The drawing under review shows one solid part. Ordinate dimensions are in mm from its lowest x, y, z. A direction names the side the tool comes from. Give positions to 0.01 mm unless a question says otherwise; leave off trailing zeros. Write each loop counter-clockwise with the first axis right and the second up, starting at its lowest first coordinate (ties: lowest second). Pieces come first, ordered by that corner, then holes. Notation, with made-up numbers: (60, 66.25) -> (65, 66.25) arc R14 ccw to (65, 91.25) -> close; hole circle Ø10 at (44, 23). An arc over 180 degrees is marked (long way). Use CSV: the item, a comma, the result in double quotes.
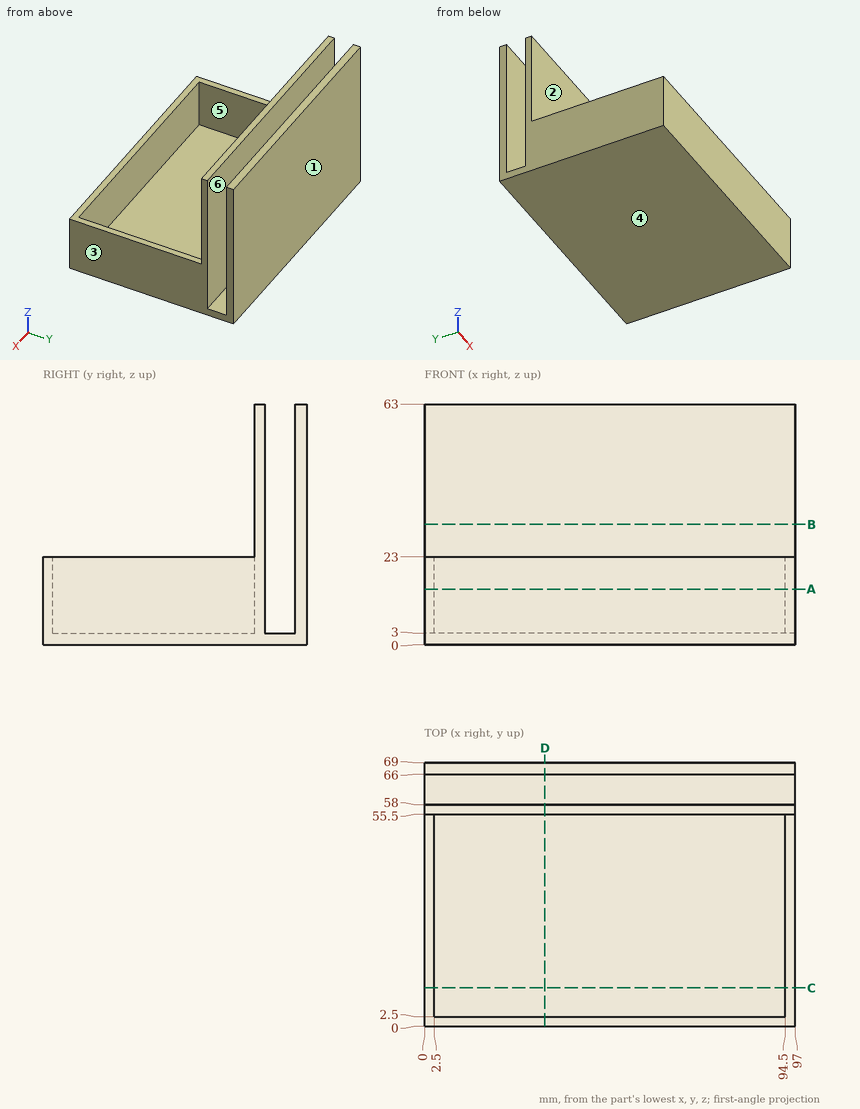
(1) Mouldability with a two-part tool opening along X and no side actions: class the marked faces 1, 2 and 3 as +X half, -X half, draft (parallel to the pull), parting line (faces both ways), or undercut.
Established:
face 1,"draft"
face 2,"undercut"
face 3,"+X half"
(2) Take a section at D-D (x = 31.5). Write out the cut boundary in (y, z).
Established:
outline,"(0, 0) -> (69, 0) -> (69, 63) -> (66, 63) -> (66, 3) -> (58, 3) -> (58, 63) -> (55.5, 63) -> (55.5, 3) -> (2.5, 3) -> (2.5, 23) -> (0, 23) -> close"
(3) Take a section at B-B (z = 31.5). Write out the cut boundary in (x, y), then the cut area to 4 significant figures.
Established:
outline,"(0, 55.5) -> (97, 55.5) -> (97, 58) -> (0, 58) -> close; (0, 66) -> (97, 66) -> (97, 69) -> (0, 69) -> close"
area,"533.5 mm2"
(4) For line 1 along Y through (x, z) = (53, 11); line 2 along Y through (x, z) = (49.5, 57); line 3 along X through (y, z) = (45, 7), list the stretches that pass through material, from the lowest coordinate up. Write a range as [from, to].
Established:
line 1,"y = [0, 2.5], [55.5, 58], [66, 69]"
line 2,"y = [55.5, 58], [66, 69]"
line 3,"x = [0, 2.5], [94.5, 97]"
(5) Clearance check with flat-ended pins moving along their axes: pin 1 (8 mm diameter, centred on x = 67.5, y = 16, fed in from +Z); pin 2 (2 mm diameter, centred on x = 84, z = 53.5, fed in from -Y). State where each tip first meets the part, or that it passes through.
Established:
pin 1,"stops at z = 3"
pin 2,"stops at y = 55.5"
(6) Take a section at A-A (z = 14.5). Write out the cut boundary in (x, y), then the cut area to 3 significant figures.
Established:
outline,"(0, 0) -> (97, 0) -> (97, 58) -> (0, 58) -> close; (0, 66) -> (97, 66) -> (97, 69) -> (0, 69) -> close; hole (2.5, 2.5) -> (94.5, 2.5) -> (94.5, 55.5) -> (2.5, 55.5) -> close"
area,"1,040 mm2"
(7) Tool access review of the marked faces 4, 5 and 6: name each direction out of +Z, -Z, +X, -X, +Y, -Y from which nothing blocks a thin tool from reaching the whole face with its end or side.
Established:
face 4,"-Z, +X, -X, +Y, -Y"
face 5,"+Z"
face 6,"+Z, +X, -X"
(8) Take a section at C-C (y = 10). Write out the cut boundary in (x, z), then the cut area to 3 significant figures.
Established:
outline,"(0, 0) -> (97, 0) -> (97, 23) -> (94.5, 23) -> (94.5, 3) -> (2.5, 3) -> (2.5, 23) -> (0, 23) -> close"
area,"391 mm2"
